Geometry check sheet. Reference: the model listing, model coordinates, mm. A direction names the side the tool comes from. Coordinates: 2 decimals unless noted, no trailing zeros. Loops run counter-clockwise (first coordinate to the right, second up) from the corner with the lowest first, then second, coordinate; pieces in that order, holes last. Notation, with made-up numbers: M 79,6.25 L 114,6.25 A34 ccw 114,45.25 Z; hole C 49,1.25 d6. An arc over 180 degrees is marked long. Use CSV: the item, a comma, the result in double quotes.
```python
from build123d import *

# Parameters (mm, degrees)
SKETCH1_R           = 85
BOSS_EXTRUDE1_DEPTH = 27
SKETCH2_R           = 10
CUT_EXTRUDE1_DEPTH  = 124.203084377
SKETCH3_R           = 8.611328572
CUT_EXTRUDE2_DEPTH  = 18.121124
CIRPATTERN1_START   = 8.878876203
CIRPATTERN1_DEPTH   = 18.121123797


# Read off the part's stored shape, not the designer's step: CirPattern1
with BuildPart() as part:
    # Sketch1 → Boss-Extrude1 (new body)
    with BuildSketch(Plane(origin=(0, 0, 0), x_dir=(1, 0, 0), z_dir=(0, 1, 0))):
        with Locations(Location((0, 0, 0), (0, 0, 270))):
            Circle(SKETCH1_R)
    extrude(amount=BOSS_EXTRUDE1_DEPTH)

    # Sketch2 → Cut-Extrude1 (cut, through all)
    with BuildSketch(Plane(origin=(0, 0, 0), x_dir=(1, 0, 0), z_dir=(0, 1, 0))):
        with Locations(Location((0, 0, 0), (0, 0, 270))):
            Circle(SKETCH2_R)
    extrude(amount=CUT_EXTRUDE1_DEPTH, mode=Mode.SUBTRACT)

    # Sketch3 → Cut-Extrude2 (cut)
    with BuildSketch(Plane(origin=(0, 27, 0), x_dir=(1, 0, 0), z_dir=(0, 1, 0))):
        with Locations((-17.200656016, 0)):
            Circle(SKETCH3_R)
    extrude(amount=-CUT_EXTRUDE2_DEPTH, mode=Mode.SUBTRACT)

    # CirPattern1 outline → CirPattern1 (cut)
    with BuildSketch(Plane(origin=(0, 0, 0), x_dir=(1, 0, 0), z_dir=(0, 1, 0)).offset(CIRPATTERN1_START)):
        with BuildLine():
            ThreePointArc((3.542234648, -9.351608081), (0, -10), (-3.542234648, -9.351608081))
            ThreePointArc((-3.542234648, -9.351608081), (-3.750765306, -9.449092341), (-3.956615815, -9.552115562))
            ThreePointArc((-3.956615815, -9.552115562), (-4.029325688, -9.333708853), (-4.107847349, -9.117323629))
            ThreePointArc((-4.107847349, -9.117323629), (-7.071067812, -7.071067812), (-9.117323629, -4.107847349))
            ThreePointArc((-9.117323629, -4.107847349), (-9.333708853, -4.029325688), (-9.552115562, -3.956615815))
            ThreePointArc((-9.552115562, -3.956615815), (-13.90524324, -7.955830216), (-19.811240963, -8.206084694))
            ThreePointArc((-19.811240963, -8.206084694), (-18.251829338, -18.251829338), (-8.206084694, -19.811240963))
            ThreePointArc((-8.206084694, -19.811240963), (0, -25.811984588), (8.206084694, -19.811240963))
            ThreePointArc((8.206084694, -19.811240963), (18.251829338, -18.251829338), (19.811240963, -8.206084694))
            ThreePointArc((19.811240963, -8.206084694), (25.811984588, 0), (19.811240963, 8.206084694))
            ThreePointArc((19.811240963, 8.206084694), (18.251829338, 18.251829338), (8.206084694, 19.811240963))
            ThreePointArc((8.206084694, 19.811240963), (0, 25.811984588), (-8.206084694, 19.811240963))
            ThreePointArc((-8.206084694, 19.811240963), (-18.251829338, 18.251829338), (-19.811240963, 8.206084694))
            ThreePointArc((-19.811240963, 8.206084694), (-13.90524324, 7.955830216), (-9.552115562, 3.956615815))
            ThreePointArc((-9.552115562, 3.956615815), (-9.333708853, 4.029325688), (-9.117323629, 4.107847349))
            ThreePointArc((-9.117323629, 4.107847349), (-7.071067812, 7.071067812), (-4.107847349, 9.117323629))
            ThreePointArc((-4.107847349, 9.117323629), (-4.029325688, 9.333708853), (-3.956615815, 9.552115562))
            ThreePointArc((-3.956615815, 9.552115562), (-3.750765306, 9.449092341), (-3.542234648, 9.351608081))
            ThreePointArc((-3.542234648, 9.351608081), (0, 10), (3.542234648, 9.351608081))
            ThreePointArc((3.542234648, 9.351608081), (3.750765306, 9.449092341), (3.956615815, 9.552115562))
            ThreePointArc((3.956615815, 9.552115562), (4.029325688, 9.333708853), (4.107847349, 9.117323629))
            ThreePointArc((4.107847349, 9.117323629), (7.071067812, 7.071067812), (9.117323629, 4.107847349))
            ThreePointArc((9.117323629, 4.107847349), (9.333708853, 4.029325688), (9.552115562, 3.956615815))
            ThreePointArc((9.552115562, 3.956615815), (9.449092341, 3.750765306), (9.351608081, 3.542234648))
            ThreePointArc((9.351608081, 3.542234648), (10, 0), (9.351608081, -3.542234648))
            ThreePointArc((9.351608081, -3.542234648), (9.449092341, -3.750765306), (9.552115562, -3.956615815))
            ThreePointArc((9.552115562, -3.956615815), (9.333708853, -4.029325688), (9.117323629, -4.107847349))
            ThreePointArc((9.117323629, -4.107847349), (7.071067812, -7.071067812), (4.107847349, -9.117323629))
            ThreePointArc((4.107847349, -9.117323629), (4.029325688, -9.333708853), (3.956615815, -9.552115562))
            ThreePointArc((3.956615815, -9.552115562), (3.750765306, -9.449092341), (3.542234648, -9.351608081))
        make_face()
    extrude(amount=CIRPATTERN1_DEPTH, mode=Mode.SUBTRACT)


solid = part.part
```
1. Section check D-D, the plane y = 6.75. Record the cut outline in (x, z), plus the area to 3 significant figures.
The answers:
outline,"C 0,0 d170; hole C 0,0 d20"
area,"22,400 mm^2"
2. Set-up check for faces 4 (the flat face through (-18, 0, -1)), 5 (the cylindrical face through (-25.81, 18.07, -0.15)): record each of +Z, -Z, +X, -X, +Y, -Y from which the full face is reachable in a straight line by a thin tool's end or side.
The answers:
face 4,"+Z, -Z, +X, -X, -Y"
face 5,"+Y"
3. Section check A-A, the plane y = 23.25. Count the separate pieces of the cut face and the enclosed holes in it, plus the area to 3 significant figures.
The answers:
separate pieces,"9"
enclosed holes,"1"
area,"20,800 mm^2"
4. Section check C-C, the plane x = 0. Record the cut outline in (y, z).
The answers:
outline,"M 0,-85 L 27,-85 L 27,-25.81 L 8.88,-25.81 L 8.88,-10 L 0,-10 Z; M 0,10 L 8.88,10 L 8.88,25.81 L 27,25.81 L 27,85 L 0,85 Z"
5. Gauge pin test, flat ends, axial feed: P1, Ø1, axis at x = 35, y = 21.5, coming from the -Z side; P2, Ø1, axis at y = 23, z = -12.5, coming from the -X side; P3, Ø2, axis at x = 51.5, y = 16, coming from the -Z side. Record the tip position at first contact, or that the pin passes through.
The answers:
P1,"z = -77.68"
P2,"x = -84.15"
P3,"z = -68.37"
6. Thickness scan on line 1 (X direction, y = 17.5, z = 0); line 2 (Z direction, x = 2, y = 12.25); line 3 (X direction, y = 19.5, z = -13). Record the ranges inside material, lowest first. Write a range as [from, to].
The answers:
line 1,"[-85, -25.81], [25.81, 85]"
line 2,"[-84.98, -25.58], [25.58, 84.98]"
line 3,"[-84, -20.73], [20.73, 84]"
7. Section check B-B, the plane z = 0. Record the cut outline in (x, y), plus the area to 3 significant figures.
The answers:
outline,"M -85,0 L -10,0 L -10,8.88 L -25.81,8.88 L -25.81,27 L -85,27 Z; M 10,0 L 85,0 L 85,27 L 25.81,27 L 25.81,8.88 L 10,8.88 Z"
area,"3,480 mm^2"
8. Release check for a two-part mould opening along X. For faces 1 (the cylindrical face through (-3.83, 7.311, 9.237)), 2 (the cylindrical face through (-51.721, 13.311, -67.453)), 3 (the flat face through (-18, 27, -20)) record: +X half, -X half, draft (parallel to the pull), parting line (faces both ways), or undercut.
The answers:
face 1,"undercut"
face 2,"parting line"
face 3,"draft"
